Can you work these out from the model? Positions are in its coordinate system, mm. Face numbers are marked on the shaded views. A direction names the side the tool comes from. Coordinates: 2 decimals unless noted, no trailing zeros. Order: outer loops, then holes, each group sorted by start corner. A loop starts at its lowest first (then second) coordinate and runs counter-clockwise, first axis right, second up. Notation, with made-up numbers: (-36.75, 89) -> (21.25, 89) arc R6 cw to (21.25, 96) -> close; hole circle Ø1 at (5.25, 16). An arc over 180 degrees is marked (long way). Use a Markdown table: item, result. Add a question column.
1. For pin 1 Ø8 at (x, y) = (8.5, 42.5) entering from -Z; pin 2 Ø1.5 at (y, z) = (17, -4.5) entering from -X; pin 3 Ø3 at (y, z) = (20, 1) entering from +X; pin 4 Ø4 at (y, z) = (26, 0) entering from -X, each with a flat end and sliding along its axis, tell me the tip position at first contact or that it passes through.
2. For the marked faces 1 and 2, which set-ups out of +Z, -Z, +X, -X, +Y, -Y let a thin tool reach every point of the face, with its end or its side?
3. Suppose I cut it at A-A, the plane y = 55. List the corners of the cut face in (x, z) for me, then the cut area to 3 significant figures.
4. If I drill on line 1 along X through (y, z) = (60.3, 0); line 2 along Y through (x, z) = (0.5, 2); line 3 along Y through (x, z) = (8.25, 5), over which ranges is the centre line in solid material (lowest first)? Write a range as from..to.
```python
from build123d import *

# Parameters (mm, degrees)
SKETCH2_R           = 10
BOSS_EXTRUDE1_DEPTH = 10
FILLET1_R           = 8
SKETCH5_R           = 0.4
SKETCH6_R           = 9
BOSS_EXTRUDE2_DEPTH = 1
CHAMFER1_SIZE       = 1
SKETCH7_R           = 1
BOSS_EXTRUDE3_DEPTH = 30
SKETCH8_R           = 0.5
CUT_EXTRUDE1_DEPTH  = 1


with BuildPart() as part:
    # Sketch2 → Boss-Extrude1 (new body)
    with BuildSketch(Plane(origin=(0, 0, 0), x_dir=(1, 0, 0), z_dir=(0, 1, 0))):
        with Locations(Location((0, 0, 0), (0, 0, 270))):
            Circle(SKETCH2_R)
    extrude(amount=BOSS_EXTRUDE1_DEPTH)

    # Loft1: read off the stored shape, not the designer's step
    # Loft1: loft between two sections, ruled curve by curve
    loft1_from = [
        Edge.make_bspline([(-12.860252555, 10, 1.901027147), (-9.058198262, 10, 27.621532257), (16.662306849, 10, 23.819477964), (12.860252555, 10, -1.901027147), (9.058198262, 10, -27.621532257), (-16.662306849, 10, -23.819477964), (-12.860252555, 10, 1.901027147)], [0, 0, 0, 0, 0.5, 0.5, 0.5, 1, 1, 1, 1], 3, [1, 0.333333333, 0.333333333, 1, 0.333333333, 0.333333333, 1]),
    ]
    loft1_to = [
        Edge.make_bspline([(-9.079588938, 30, -4.190592406), (-17.460773749, 30, 13.968585471), (0.698404127, 30, 22.349770282), (9.079588938, 30, 4.190592406), (17.460773749, 30, -13.968585471), (-0.698404127, 30, -22.349770282), (-9.079588938, 30, -4.190592406)], [0, 0, 0, 0, 0.5, 0.5, 0.5, 1, 1, 1, 1], 3, [1, 0.333333333, 0.333333333, 1, 0.333333333, 0.333333333, 1]),
    ]
    loft1 = Solid(Shell([*[Face.make_surface_from_curves(loft1_from[k], loft1_to[k]) for k in range(1)], Face(Wire(loft1_from)), Face(Wire(loft1_to))]))
    add(loft1)

    # Fillet1
    # the kernel refuses this fillet: 8 mm, written as the material it takes off along each edge
    with BuildSketch(Plane(origin=(0, 10, 0), x_dir=(-0.9892501965607676, 0, 0.14623285747219308), z_dir=(-0.14623285747219308, 0, -0.9892501965607676))) as fillet1_piece_1:
        with BuildLine():
            CenterArc((3.770111358, 5.018813356), FILLET1_R, 321.144997334, 49.449726364)
            Line((10, 0), (10.124597773, -0.100376267))
            ThreePointArc((10.124597773, -0.100376267), (11.5, -0.16), (13, -0.16))
            Line((13, -0.16), (13.155876196, 0.036091708))
            ThreePointArc((13.155876196, 0.036091708), (12.43891649, 3.270626899), (11.791002002, 6.519117749))
            Line((11.791002002, 6.519117749), (11.633729636, 6.489700016))
        make_face()
    revolve(axis=Axis((0, 10, 0), (0, 1, 0)), mode=Mode.SUBTRACT)

    # Sketch5 → Cut-Revolve1 (revolve, cut)
    with BuildSketch(Plane(origin=(0, 0, 0), x_dir=(0, 0, -1), z_dir=(1, 0, 0))):
        with Locations((-11.633729637, 16.489700016)):
            Circle(SKETCH5_R)
    revolve(axis=Axis((0, 16.489700016, 0), (0, 1, 0)), mode=Mode.SUBTRACT)

    # Sketch6 → Boss-Extrude2 (add)
    with BuildSketch(Plane(origin=(0, 30, 0), x_dir=(1, 0, 0), z_dir=(0, 1, 0))):
        with Locations(Location((0, 0, 0), (0, 0, 270))):
            Circle(SKETCH6_R)
    extrude(amount=BOSS_EXTRUDE2_DEPTH)

    # Chamfer1
    chamfer1_edges = [part.edges().sort_by_distance(p)[0] for p in [
        (0, 31, -9),
    ]]
    chamfer(chamfer1_edges, length=CHAMFER1_SIZE - 0.0001)  # a hair under: the kernel refuses the full size

    # Sketch7 → Boss-Extrude3 (add)
    with BuildSketch(Plane(origin=(0, 31, 0), x_dir=(1, 0, 0), z_dir=(0, 1, 0))):
        with Locations(Location((0, 0, 0), (0, 0, 270))):
            Circle(SKETCH7_R)
    extrude(amount=BOSS_EXTRUDE3_DEPTH)

    # Sketch8 → Cut-Extrude1 (cut)
    with BuildSketch(Plane(origin=(0, 61, 0), x_dir=(1, 0, 0), z_dir=(0, 1, 0))):
        with Locations(Location((0, 0, 0), (0, 0, 270))):
            Circle(SKETCH8_R)
    extrude(amount=-CUT_EXTRUDE1_DEPTH, mode=Mode.SUBTRACT)


solid = part.part
```
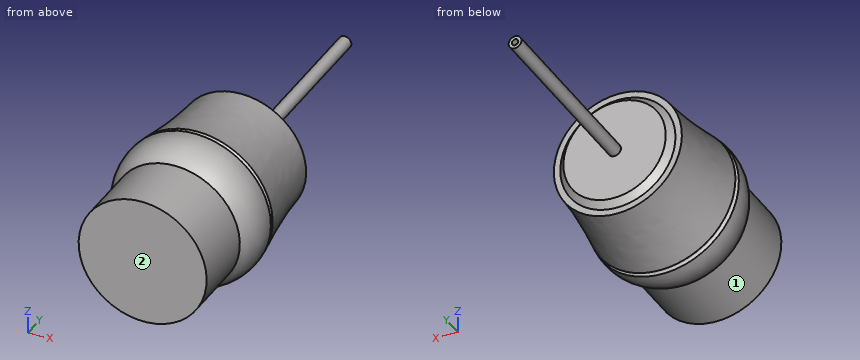
Worked out:
| question | item | result |
|---|---|---|
| 1 | pin 1 | passes through |
| 1 | pin 2 | stops at x = -10.93 |
| 1 | pin 3 | stops at x = 11.25 |
| 1 | pin 4 | stops at x = -10.48 |
| 2 | face 1 | -Y |
| 2 | face 2 | +Z, -Z, +X, -X, -Y |
| 3 | outline | circle Ø2 at (0, 0) |
| 3 | area | 3.14 mm² |
| 4 | line 1 | x = -1..-0.5, 0.5..1 |
| 4 | line 2 | y = 0..31 |
| 4 | line 3 | y = 0..30 |
